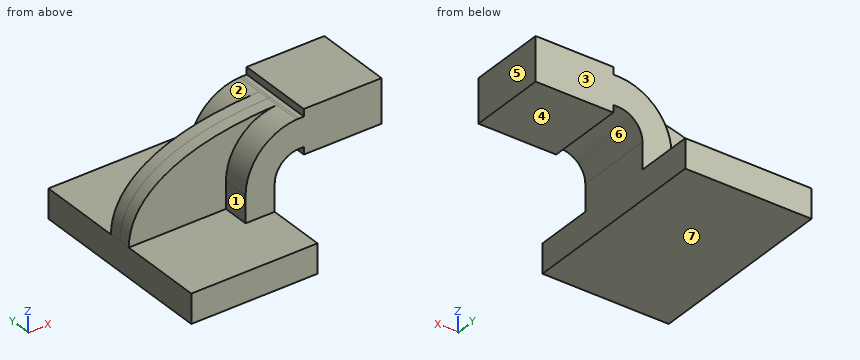
from build123d import *

# Parameters (mm, degrees)
F1_DEPTH = 63.5
F2_DEPTH = 25.4
F3_DEPTH = 7.9375


with BuildPart() as f1:
    # F0 (on Front) → F1 (new body, symmetric)
    with BuildSketch(Plane.XZ):
        Polygon((22.225, 9.525), (-41.275, 9.525), (-41.275, -9.525), (41.275, -9.525), (41.275, 9.525), align=None)
    extrude(amount=F1_DEPTH, both=True)

    # F0 (on Front) → F2 (join, symmetric)
    with BuildSketch(Plane.XZ):
        Polygon((60.325, 66.675), (60.325, 61.9252), (60.325, 42.8752), (60.325, 38.1), (111.125, 38.1), (111.125, 66.675), align=None)
        with BuildLine():
            Line((22.225, 27.0002), (22.225, 9.525))
            Line((22.225, 9.525), (41.275, 9.525))
            Line((41.275, 9.525), (41.275, 27.0002))
            ThreePointArc((41.275, 27.0002), (45.92468, 38.22552), (57.15, 42.8752))
            Line((57.15, 42.8752), (60.325, 42.8752))
            Line((60.325, 42.8752), (60.325, 61.9252))
            Line((60.325, 61.9252), (57.15, 61.9252))
            add(Edge.make_bspline(
                [(55.648092, 61.892891), (56.146402, 61.904771), (56.647035, 61.915543), (57.15, 61.9252)],
                knots=[110.762512, 110.762512, 110.762512, 110.762512, 111.504536, 111.504536, 111.504536, 111.504536], degree=3))
            ThreePointArc((55.648092, 61.892891), (31.92888, 51.159065), (22.225, 27.0002))
        make_face()
    extrude(amount=F2_DEPTH, both=True)

    # F0 (on Front) → F3 (join, symmetric)
    with BuildSketch(Plane.XZ):
        with BuildLine():
            add(Edge.make_bspline(
                [(-41.275, 9.525), (-41.346803, 33.675018), (-18.734938, 60.119621), (55.648092, 61.892891)],
                knots=[0, 0, 0, 0, 110.762512, 110.762512, 110.762512, 110.762512], degree=3))
            Line((-41.275, 9.525), (22.225, 9.525))
            Line((22.225, 9.525), (22.225, 27.0002))
            ThreePointArc((22.225, 27.0002), (31.92888, 51.159065), (55.648092, 61.892891))
        make_face()
    extrude(amount=F3_DEPTH, both=True)


solid = f1.part
Check sheet for the modelled part. Datum: model origin and axes. Units: mm. Face numbers are marked on the shaded views. A direction names the side the tool comes from. Give positions to 0.01 mm unless a question says otherwise; leave off trailing zeros. Write each loop counter-clockwise with the first axis right and the second up, starting at its lowest first coordinate (ties: lowest second). Pieces come first, ordered by that corner, then holes. Notation, with made-up numbers: (-37, 47.5) -> (3, 47.5) arc R27 cw to (3, 74.5) -> close; hole circle Ø9 at (-7.5, -26). An arc over 180 degrees is marked (long way). One line per item, written item: value. Start each with the question number.
Item 1: Section check B-B on y = 55. Record the cut outline in (x, z) (3 decimals), then the cut area to 3 significant figures.
Item 2: Draft check along X on the marked faces 5, 6 and 7. Enter one of: +X half, -X half, draft (parallel to the pull), parting line (faces both ways), or undercut.
Item 3: Gauge pin test, flat ends, axial feed: pin 1 (2.5 mm diameter, centred on y = -7.5, z = 64.5, fed in from -X) (3 decimals); pin 2 (4 mm diameter, centred on y = 12, z = 39.5, fed in from -X); pin 3 (2.5 mm diameter, centred on x = 59, y = 10.5, fed in from -Z). Record the tip position at first contact, or that the pin passes through.
Item 4: Section check A-A on z = 1. Record the cut outline in (x, y) (3 decimals), then the cut area to 3 significant figures.
Item 5: Tool access check on the marked faces 1, 2, 3 and 4. Record the directions out of +Z, -Z, +X, -X, +Y, -Y that give a thin tool (end or side, any length) a straight path to the whole face; none if there is none.
Item 6: Material ranges on probe 1 along Z at (x, y) = (98, 7.5) (3 decimals); probe 2 along Y at (x, z) = (-20.5, 43); probe 3 along X at (y, z) = (-2.5, 39) (3 decimals), recorded low to high. Write a range as from..to.
Results list:
1. outline: (-41.275, -9.525) -> (41.275, -9.525) -> (41.275, 9.525) -> (-41.275, 9.525) -> close
1. area: 1,570 mm²
2. face 5: +X half
2. face 6: undercut
2. face 7: draft
3. pin 1: x = 60.325
3. pin 2: x = 23.84
3. pin 3: z = 42.88
4. outline: (-41.275, -63.5) -> (41.275, -63.5) -> (41.275, 63.5) -> (-41.275, 63.5) -> close
4. area: 10,500 mm²
5. face 1: +Z, -X, -Y
5. face 2: +Z, -X, +Y
5. face 3: +Z, +X, -X, +Y
5. face 4: -Z, +X, +Y, -Y
6. probe 1: 38.1..66.675
6. probe 2: -7.94..7.94
6. probe 3: -27.398..46.757, 60.325..111.125
